Can you work these out from the drawing? Everything is in mm from the part's minimum corner. Coordinates: 2 decimals unless noted, no trailing zeros. Loops run counter-clockwise (first coordinate to the right, second up) from the corner with the lowest first, then second, coordinate; pieces in that order, holes last. Notation, with made-up numbers: (-10, 65) -> (36, 65) arc R6 ccw to (36, 70) -> close; hole circle Ø6 at (46.5, 61). An arc over 180 degrees is marked (long way). One line per question, with ' | ' between items.
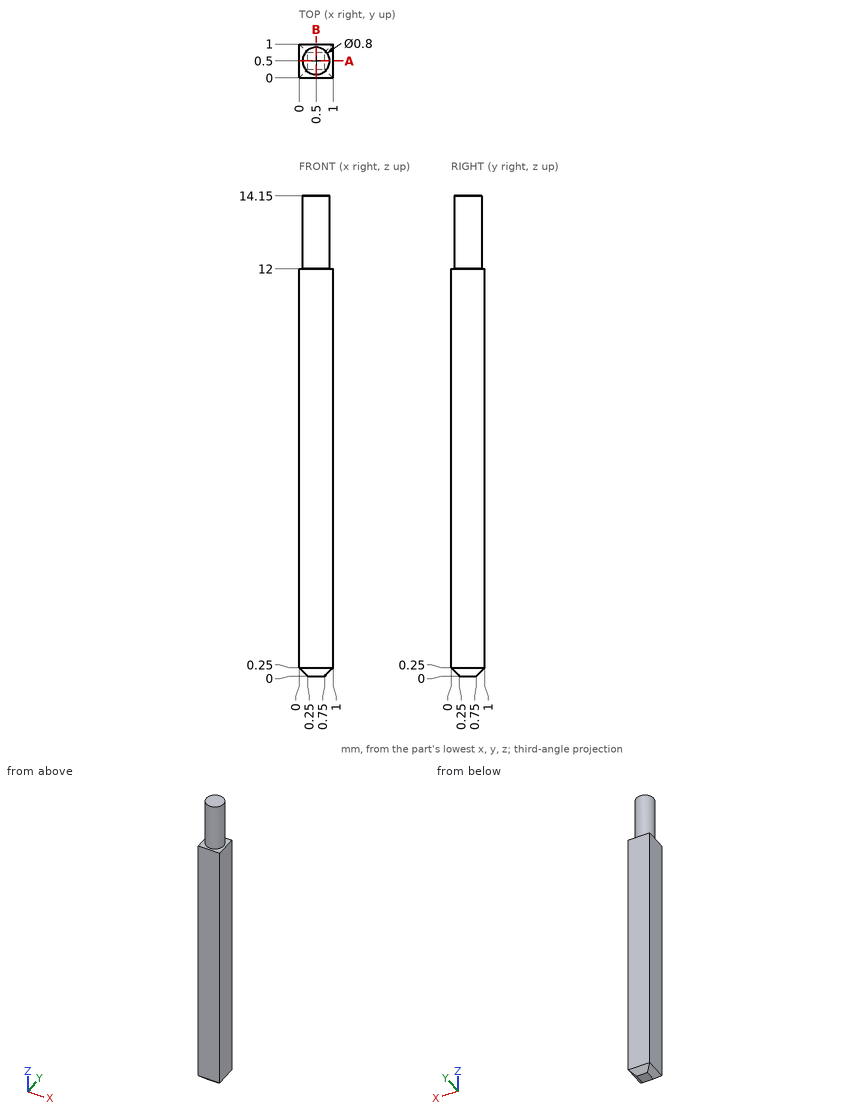
Q1. Please list where these lines run through material, in increasing order: L1, parallel to Z at x = 0.85, y = 0.6; L2, parallel to Z at x = 0.9, y = 0.85; L3, parallel to Y at x = 0.2, z = 13.75. Write a range as [from, to].
Values follow:
L1: z = [0.1, 14.15] | L2: z = [0.15, 12] | L3: y = [0.24, 0.76]
Q2. Imagine slicing it at A-A on y = 0.5. Write out the boundary of the cut face in (x, z), plus the area to 3 significant figures.
Values follow:
outline: (0, 0.25) -> (0.25, 0) -> (0.75, 0) -> (1, 0.25) -> (1, 12) -> (0.9, 12) -> (0.9, 14.15) -> (0.1, 14.15) -> (0.1, 12) -> (0, 12) -> close | area: 13.7 mm2
